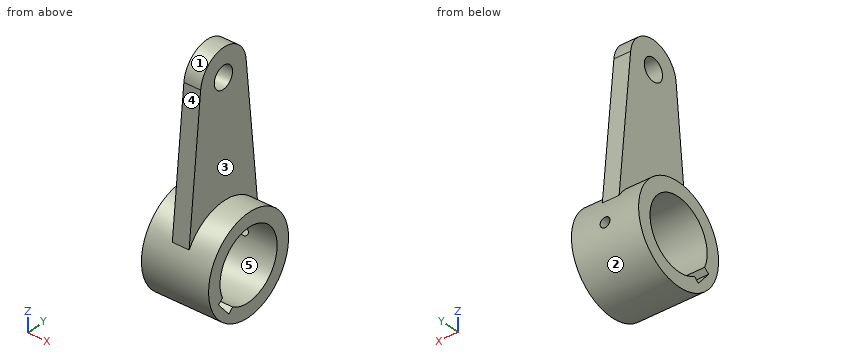
```python
from build123d import *

# Parameters (mm, degrees)
SKETCH1_R           = 35
SKETCH1_R_2         = 25
BOSS_EXTRUDE1_DEPTH = 24
BOSS_EXTRUDE2_DEPTH = 6
SKETCH3_R           = 8
CUT_EXTRUDE1_DEPTH  = 15
CUT_EXTRUDE2_DEPTH  = 150.875815261
SKETCH6_R           = 3.5
CUT_EXTRUDE3_DEPTH  = 24


with BuildPart() as part:
    # Sketch1 → Boss-Extrude1 (new, symmetric)
    with BuildSketch(Plane(origin=(0, 0, 0), x_dir=(0, 0, -1), z_dir=(1, 0, 0))):
        Circle(SKETCH1_R)
        Circle(SKETCH1_R_2, mode=Mode.SUBTRACT)
    extrude(amount=BOSS_EXTRUDE1_DEPTH, both=True)

    # Sketch2 → Boss-Extrude2 (add, symmetric)
    with BuildSketch(Plane(origin=(0, 0, 0), x_dir=(0, 0, -1), z_dir=(1, 0, 0))):
        with BuildLine():
            Line((-18.027756377, 30), (-119.579019246, 19.901846216))
            ThreePointArc((-119.579019246, 19.901846216), (-137.6, 0), (-119.579019246, -19.901846216))
            Line((-119.579019246, -19.901846216), (-18.027756377, -30))
            ThreePointArc((-18.027756377, -30), (-35, 0), (-18.027756377, 30))
        make_face()
    extrude(amount=BOSS_EXTRUDE2_DEPTH, both=True)

    # Sketch3 → Cut-Extrude1 (cut)
    with BuildSketch(Plane(origin=(6, 0, 0), x_dir=(0, 0, -1), z_dir=(1, 0, 0))):
        with Locations((-117.6, 0)):
            Circle(SKETCH3_R)
    extrude(amount=-CUT_EXTRUDE1_DEPTH, mode=Mode.SUBTRACT)

    # Sketch5 → Cut-Extrude2 (cut, through all)
    with BuildSketch(Plane(origin=(24, 0, 0), x_dir=(0, 0, -1), z_dir=(1, 0, 0))):
        Polygon((23.681757978, -17.332753361), (12.957135774, -26.331779897), (3.997953594, -15.654642346), (14.722575797, -6.655615811), align=None)
    extrude(amount=-CUT_EXTRUDE2_DEPTH, mode=Mode.SUBTRACT)

    # Sketch6 → Cut-Extrude3 (cut)
    with BuildSketch(Plane(origin=(0, 35, 0), x_dir=(-1, 0, 0), z_dir=(0, 1, 0))):
        with Locations(Location((0, 0, 0), (0, 0, 90))):
            Circle(SKETCH6_R)
    extrude(amount=-CUT_EXTRUDE3_DEPTH, mode=Mode.SUBTRACT)


solid = part.part
```
Source: CAD feature listing. Evaluate the final solid. Frame: model axes, mm. Face numbers are marked on the shaded views. A direction names the side the tool comes from. Coordinates: 2 decimals unless noted, no trailing zeros. Write each loop counter-clockwise with the first axis right and the second up, starting at its lowest first coordinate (ties: lowest second). Pieces come first, ordered by that corner, then holes. Notation, with made-up numbers: (-17.5, 45.5) -> (18.5, 45.5) arc R25 cw to (18.5, 61.5) -> close; hole circle Ø1 at (1, 39.5). An arc over 180 degrees is marked (long way). Return JSON: item names as keys, results as strings. Group by question number.
1) Section query C-C, the plane y = -11.5. Return loops of the section in (x, z), plus the area to 3 significant figures.
2) Ray query, line 1 along Y through (x, z) = (10, 0); line 2 along X through (y, z) = (21.5, 98.5). Return the intervals inside material, ascending.
3) Contact query for flat-ended pins moving along their axis: P1, Ø18, axis at y = 4, z = 98, coming from the +X side; P2, Ø10, axis at x = -14, y = -15.5, coming from the +Z side; P3, Ø3, axis at x = -1.5, z = 101.5, coming from the +Y side. Output: stop coordinate, or through.
4) Set-up query: the marked faces 1 and 2. Return all of +Z, -Z, +X, -X, +Y, -Y with unobstructed straight access to the full face (end or side cutting, diameter ignored); none if empty.
5) Section query B-B, the plane y = 0. Return loops of the section in (x, z), plus the area to 3 significant figures.
6) Section query A-A, the plane z = 0. Return loops of the section in (x, y), plus the area to 3 significant figures.
7) Mould query, pull axis Y, two halves, no side actions, for the marked faces 3, 4 and 5. Classes: +Y half, -Y half, draft (parallel to the pull), parting line (faces both ways), or undercut.
8) Section query D-D, the plane x = 0. Return loops of the section in (y, z), plus the area to 3 significant figures.
From the geometry:
{
 "1": {"outline": "(-24, -33.06) -> (24, -33.06) -> (24, -22.2) -> (-24, -22.2) -> close; (-24, 22.2) -> (24, 22.2) -> (24, 33.06) -> (6, 33.06) -> (6, 133.96) -> (-6, 133.96) -> (-6, 33.06) -> (-24, 33.06) -> close", "area": "2,250 mm²"},
 "2": {"line 1": "-35 to -25, 25 to 35", "line 2": "-6 to 6"},
 "3": {"P1": "x = 6", "P2": "z = 33.39", "P3": "y = 21.85"},
 "4": {"face 1": "+Z, +X, -X", "face 2": "none"},
 "5": {"outline": "(-24, -35) -> (24, -35) -> (24, -25) -> (-24, -25) -> close; (-24, 25) -> (24, 25) -> (24, 35) -> (6, 35) -> (6, 109.6) -> (-6, 109.6) -> (-6, 35) -> (-24, 35) -> close; (-6, 125.6) -> (6, 125.6) -> (6, 137.6) -> (-6, 137.6) -> close", "area": "2,000 mm²"},
 "6": {"outline": "(-24, -35) -> (24, -35) -> (24, -25) -> (-24, -25) -> close; (-24, 25) -> (-3.5, 25) -> (-3.5, 35) -> (-24, 35) -> close; (3.5, 25) -> (24, 25) -> (24, 35) -> (3.5, 35) -> close", "area": "890 mm²"},
 "7": {"face 3": "draft", "face 4": "-Y half", "face 5": "undercut"},
 "8": {"outline": "(-30, 18.03) arc R35 ccw (long way) to (34.82, -3.5) -> (24.75, -3.5) arc R25 cw to (-13.89, -20.79) -> (-17.33, -23.68) -> (-26.33, -12.96) -> (-22.88, -10.06) arc R25 cw (long way) to (24.75, 3.5) -> (34.82, 3.5) arc R35 ccw to (30, 18.03) -> (19.9, 119.58) arc R20 ccw to (-19.9, 119.58) -> close; hole circle Ø16 at (0, 117.6)", "area": "6,460 mm²"}
}
